Here's how the part is built. I have some questions about the finished solid (model axes, mm). A direction names the side the tool comes from. Round coordinates to 2 decimals unless told otherwise and drop trailing zeros. Order: outer loops, then holes, each group sorted by start corner. A loop starts at its lowest first (then second) coordinate and runs counter-clockwise, first axis right, second up. Notation, with made-up numbers: M 14.5,33.5 L 55.5,33.5 A19 cw 55.5,47.5 Z; hole C 72.25,65.5 d8. An arc over 180 degrees is marked long. Write each question's results on one line, items separated by ' | '. Start each with the question number.
```python
from build123d import *

# Parameters (mm, degrees)
SKETCH1_R                      = 12.7
BOSS_EXTRUDE1_DEPTH            = 10
SKETCH2_R                      = 8.5
BOSS_EXTRUDE2_DEPTH            = 3
F_5_5_5_5_DIAMETER_HOLE1_D     = 5.5
F_6_3_6_3_DIAMETER_HOLE1_D     = 6.3
F_6_3_6_3_DIAMETER_HOLE1_DEPTH = 12
F_6_3_6_3_DIAMETER_HOLE1_TIP   = 1.89271095
F_1_5MM_DOWEL_HOLE1_D          = 1.5
F_1_5MM_DOWEL_HOLE1_DEPTH      = 3
F_1_5MM_DOWEL_HOLE1_TIP        = 0.450645464


with BuildPart() as part:
    # Sketch1 → Boss-Extrude1 (new body)
    with BuildSketch(Plane(origin=(0, 0, 0), x_dir=(1, 0, 0), z_dir=(0, 1, 0))):
        Circle(SKETCH1_R)
    extrude(amount=BOSS_EXTRUDE1_DEPTH)

    # Sketch2 → Boss-Extrude2 (add)
    with BuildSketch(Plane(origin=(0, 10, 0), x_dir=(1, 0, 0), z_dir=(0, 1, 0))):
        Circle(SKETCH2_R)
    extrude(amount=BOSS_EXTRUDE2_DEPTH)

    # Ø5.5 (5.5) Diameter Hole1 (through all)
    with Locations(Plane(origin=(0, 0, 0), x_dir=(-1, 0, 0), z_dir=(0, -1, 0))):
        with Locations((0, 0)):
            Hole(F_5_5_5_5_DIAMETER_HOLE1_D / 2)

    # Ø6.3 (6.3) Diameter Hole1
    with Locations(Plane(origin=(0, 0, 0), x_dir=(-1, 0, 0), z_dir=(0, -1, 0))):
        with Locations((0, 0)):
            Hole(F_6_3_6_3_DIAMETER_HOLE1_D / 2, depth=F_6_3_6_3_DIAMETER_HOLE1_DEPTH)
            with Locations((0, 0, -(F_6_3_6_3_DIAMETER_HOLE1_DEPTH + F_6_3_6_3_DIAMETER_HOLE1_TIP / 2))):  # 118° drill point
                Cone(0, F_6_3_6_3_DIAMETER_HOLE1_D / 2, F_6_3_6_3_DIAMETER_HOLE1_TIP, mode=Mode.SUBTRACT)

    # Ø1.5mm Dowel Hole1
    with Locations(Plane(origin=(0, 10, 0), x_dir=(1, 0, 0), z_dir=(0, 1, 0))):
        with Locations((0, 10.5), (0, -10.5)):
            Hole(F_1_5MM_DOWEL_HOLE1_D / 2, depth=F_1_5MM_DOWEL_HOLE1_DEPTH)
            with Locations((0, 0, -(F_1_5MM_DOWEL_HOLE1_DEPTH + F_1_5MM_DOWEL_HOLE1_TIP / 2))):  # 118° drill point
                Cone(0, F_1_5MM_DOWEL_HOLE1_D / 2, F_1_5MM_DOWEL_HOLE1_TIP, mode=Mode.SUBTRACT)


solid = part.part
```
(1) If we mould it in two halves opening along Z, with no side actions, what happens to faces 4 (the conical face through (0.07, 6.63, -10.61)), 5 (the flat face through (3, 0, 3)), 6 (the cylindrical face through (0.098, 8.479, -11.244)), 7 (the cylindrical face through (4.57, 11.479, -7.167))? For each: pulls with the +Z half, pulls with the -Z half, needs draft (parallel to the pull), parting line crosses it, or undercut.
(2) I want a section at C-C on y = 8. Write out the boundary of the cut face in (x, z).
(3) I want a section at B-B on y = 5.5. Write out the boundary of the cut face in (x, z), and give its area (3 significant figures).
(4) I want a section at D-D on z = 5.75. Write out the boundary of the cut face in (x, y).
(5) Please list where these lines run through material, in increasing order: line 1 (Z direction, x = 0, y = 8.05); line 2 (X direction, y = 7.8, z = -10.5); line 3 (Z direction, x = 0, y = 3.75).
(6) I'm going to push flat-ended pins straight in: pin 1 Ø5 at (x, z) = (0, 0) entering from +Y; pin 2 Ø0.9 at (x, z) = (0, -10.5) entering from +Y; pin 3 Ø3 at (x, y) = (-4, 4.5) entering from -Z; pin 4 Ø4 at (x, y) = (9.5, 8) entering from -Z. Where does each tip first touch, or does it pass through?
(7) I want a section at A-A on z = 0. Write out the boundary of the cut face in (x, y), and give its area (3 significant figures).
(8) On a 3-axis mill with a long thin cutter (end or side, diameter ignored), from which of +Z, -Z, +X, -X, +Y, -Y can I reach the whole of each face in a straight line? I mean faces 1 (the cylindrical face through (-2.5, 6.084, 1.917)), 2 (the flat face through (8.3, 10, 2.6)), 3 (the cylindrical face through (-2.75, 4.93, 12.4)). Say none if no direction works.
Solutions:
1) face 4: undercut | face 5: needs draft | face 6: undercut | face 7: parting line crosses it
2) outline: C 0,0 d25.4; hole C 0,0 d6.3; hole C 0,-10.5 d1.5; hole C 0,10.5 d1.5
3) outline: C 0,0 d25.4; hole C 0,0 d6.3 | area: 476 mm^2
4) outline: M -11.32,0 L 11.32,0 L 11.32,10 L 6.26,10 L 6.26,13 L -6.26,13 L -6.26,10 L -11.32,10 Z
5) line 1: -12.7 to -11.25, -9.75 to -3.15, 3.15 to 9.75, 11.25 to 12.7 | line 2: -7.14 to -0.75, 0.75 to 7.14 | line 3: -12.7 to -3.15, 3.15 to 12.7
6) pin 1: through | pin 2: y = 6.82 | pin 3: z = -12.45 | pin 4: z = -10.25
7) outline: M -12.7,0 L -3.15,0 L -3.15,12 L -2.75,12.24 L -2.75,13 L -8.5,13 L -8.5,10 L -12.7,10 Z; M 2.75,12.24 L 3.15,12 L 3.15,0 L 12.7,0 L 12.7,10 L 8.5,10 L 8.5,13 L 2.75,13 Z | area: 224 mm^2
8) face 1: -Y | face 2: +Y | face 3: +Y, -Y
